from build123d import *

# Parameters (mm, degrees)
F0_W      = 76.2
F0_H      = 101.6
F1_DEPTH  = 25.4
F2_R      = 15.875
F3_SIZE   = 5.08
F4_R      = 6.35
F5_DEPTH  = 25.4
F6_W      = 66.04
F6_H      = 19.05
F7_DEPTH  = 38.1
F9_DEPTH  = 19.05
F10_R     = 9.525
F11_DEPTH = 25.4
F13_DEPTH = 25.4
F14_R     = 6.35


with BuildPart() as f1:
    # F0 (on Top) → F1 (new body)
    with BuildSketch(Plane.XY):
        with Locations((18.6636974156, 4.0336294651)):
            Rectangle(F0_W, F0_H)
    extrude(amount=F1_DEPTH)

    # F2
    f2_edges = [f1.edges().sort_by_distance(p)[0] for p in [
        (-19.436303, -46.766371, 12.7),
        (56.763697, -46.766371, 12.7),
        (56.763697, 54.833629, 12.7),
        (-19.436303, 54.833629, 12.7),
    ]]
    fillet(f2_edges, radius=F2_R)

    # F3
    f3_edges = [f1.edges().sort_by_distance(p)[0] for p in [
        (18.663697, 54.833629, 25.4),
        (-14.786623, 50.18395, 25.4),
        (-19.436303, 4.033629, 25.4),
        (-14.786623, -42.116691, 25.4),
        (18.663697, -46.766371, 25.4),
        (52.114018, -42.116691, 25.4),
        (56.763697, 4.033629, 25.4),
        (52.114018, 50.18395, 25.4),
    ]]
    chamfer(f3_edges, length=F3_SIZE)

    # F4 (on face) → F5 (cut)
    with BuildSketch(Plane.XY.offset(25.4)):
        with Locations((-3.5613025844, -30.8913705349)):
            Circle(F4_R)
        with Locations((-3.5613025844, 38.9586294651)):
            Circle(F4_R)
        with Locations((40.8886974156, 38.9586294651)):
            Circle(F4_R)
        with Locations((40.8886974156, -30.8913705349)):
            Circle(F4_R)
    extrude(amount=-F5_DEPTH, mode=Mode.SUBTRACT)

    # F6 (on face) → F7 (join)
    with BuildSketch(Plane.XY.offset(25.4)):
        with Locations((18.6636974156, 13.5586294651)):
            Rectangle(F6_W, F6_H)
    extrude(amount=F7_DEPTH)

    # F8 (on face) → F9 (join)
    with BuildSketch(Plane.XZ.offset(-4.0336294651)):
        with BuildLine():
            Line((-14.3563025844, 63.5), (51.6836974156, 63.5))
            ThreePointArc((51.6836974156, 63.5), (18.6636974156, 94.0767991723), (-14.3563025844, 63.5))
        make_face()
    extrude(amount=-F9_DEPTH)

    # F10 (on face) → F11 (cut)
    with BuildSketch(Plane.XZ.offset(-4.0336294651)):
        with Locations((18.6636974156, 63.5)):
            Circle(F10_R)
    extrude(amount=-F11_DEPTH, mode=Mode.SUBTRACT)

    # F12 (on face) → F13 (cut)
    with BuildSketch(Plane.XZ.offset(-4.0336294651)):
        Polygon((9.1407453584, 94.5832133293), (9.1407453584, 63.5), (28.1886974156, 63.5), (28.2250996679, 63.5), (28.2250996679, 94.5832133293), align=None)
    extrude(amount=-F13_DEPTH, mode=Mode.SUBTRACT)

    # F14
    f14_edges = [f1.edges().sort_by_distance(p)[0] for p in [
        (18.663697, 4.033629, 25.4),
        (18.663697, 23.083629, 25.4),
    ]]
    fillet(f14_edges, radius=F14_R)


solid = f1.part
Design review of the part built by this model. Coordinates are the model's own, in mm. A direction names the side the tool comes from. Give positions to 0.01 mm unless a question says otherwise; leave off trailing zeros. Loops run counter-clockwise (first coordinate to the right, second up) from the corner with the lowest first, then second, coordinate; pieces in that order, holes last. Notation, with made-up numbers: (-30.5, -22) -> (-10.5, -22) arc R12 cw to (-10.5, -13) -> close; hole circle Ø7 at (45, 45.25). An arc over 180 degrees is marked (long way). One line per question, with ' | ' between items. Start each with the question number.
(1) Draft analysis for pull direction X (two halves, no side actions). For faces 5 (the face through (26, 23.084, 56)), 6 (the face through (9.141, 13, 78)), 7 (the face through (54.259, 4.523, 22.824)), state which applies: +X half, -X half, draft (parallel to the pull), parting line (faces both ways), or undercut.
(2) We need section C-C (x = 37). State the section outline as (y, z) points, and give its area (3 significant figures).
(3) For faces 1 (the face through (28.225, 13, 78)), 2 (the face through (18, -22, 25.4)), 3 (the face through (52.2, 50.1, 10.3)), 4 (the face through (51.684, 13, 44)), list the 3-axis set-ups (+Z, -Z, +X, -X, +Y, -Y) from which the entire face can be reached by the end or side of a thin tool; tool diameter is ignored.
(4) We need section A-A (z = 11). State the section outline as (x, y) points (3 decimals).
(5) We need section B-B (y = -26.5). State the section outline as (x, z) points, and give its area (3 significant figures).
(6) Insertion check: P1, Ø16.5, axis at x = -3.56, y = 38.96, coming from the -Z side; P2, Ø20.5, axis at x = 40.89, y = -30.89, coming from the +Z side; P3, Ø1.5, axis at x = 44.5, z = 30, coming from the -Y side; P4, Ø6, axis at x = 25, z = 40.5, coming from the +Y side. Each pin has a flat end and moves straight along its axis. Give the tip position at first contact, or say it passes through.
(7) For line 1 (Y direction, x = 46, z = 16); line 2 (Z direction, x = 2, y = -19); line 3 (Y direction, x = 50, z = 32), list the stretches that pass through material, from the lowest coordinate up.
The answers:
1) face 5: draft | face 6: undercut | face 7: +X half
2) outline: (-46.77, 0) -> (-35.91, 0) -> (-35.91, 25.4) -> (-41.69, 25.4) -> (-46.77, 20.32) -> close; (-25.87, 0) -> (33.94, 0) -> (33.94, 25.4) -> (29.43, 25.4) arc R6.35 cw to (23.08, 31.75) -> (23.08, 88.54) -> (4.03, 88.54) -> (4.03, 31.75) arc R6.35 cw to (-2.32, 25.4) -> (-25.87, 25.4) -> close; (43.98, 0) -> (54.83, 0) -> (54.83, 20.32) -> (49.75, 25.4) -> (43.98, 25.4) -> close | area: 3,260 mm^2
3) face 1: +Z, +Y, -Y | face 2: +Z, +X, -X, -Y | face 3: +Z, -Z, +X, +Y | face 4: +Z, +X, +Y, -Y
4) outline: (-19.436, -30.891) arc R15.875 ccw to (-3.561, -46.766) -> (40.889, -46.766) arc R15.875 ccw to (56.764, -30.891) -> (56.764, 38.959) arc R15.875 ccw to (40.889, 54.834) -> (-3.561, 54.834) arc R15.875 ccw to (-19.436, 38.959) -> close; hole circle Ø12.7 at (-3.561, -30.891); hole circle Ø12.7 at (-3.561, 38.959); hole circle Ø12.7 at (40.889, -30.891); hole circle Ø12.7 at (40.889, 38.959)
5) outline: (-19.44, 0) -> (-8.15, 0) -> (-8.15, 25.4) -> (-14.36, 25.4) -> (-19.44, 20.32) -> close; (1.03, 0) -> (36.3, 0) -> (36.3, 25.4) -> (1.03, 25.4) -> close; (45.48, 0) -> (56.76, 0) -> (56.76, 20.32) -> (51.68, 25.4) -> (45.48, 25.4) -> close | area: 1,440 mm^2
6) P1: stops at z = 0 | P2: stops at z = 25.4 | P3: stops at y = 3.52 | P4: stops at y = 23.08
7) line 1: y = -45.92 to -34.66, -27.12 to 35.19, 42.73 to 53.99 | line 2: z = 0 to 25.4 | line 3: y = 4.03 to 23.08
